```python
from build123d import *

# Parameters (mm, degrees)
F0_R     = 9
F0_R_2   = 9.5
F1_DEPTH = 3
F3_DEPTH = 6.001


with BuildPart() as f1:
    # F0 (on Top) → F1 (new body, symmetric)
    with BuildSketch(Plane.XY):
        with BuildLine():
            Line((22.5, 12.5), (-22.5, 12.5))
            ThreePointArc((-22.5, 12.5), (-31.338835, 8.838835), (-35, 0))
            ThreePointArc((-35, 0), (-31.338835, -8.838835), (-22.5, -12.5))
            Line((-22.5, -12.5), (22.5, -12.5))
            ThreePointArc((22.5, -12.5), (31.338835, -8.838835), (35, 0))
            ThreePointArc((35, 0), (31.338835, 8.838835), (22.5, 12.5))
        make_face()
        with Locations((-22.5, 0)):
            Circle(F0_R, mode=Mode.SUBTRACT)
        Circle(F0_R_2, mode=Mode.SUBTRACT)
        with Locations((22.5, 0)):
            Circle(F0_R, mode=Mode.SUBTRACT)
    extrude(amount=F1_DEPTH, both=True)

    # F2 (on face) → F3 (cut, through all)
    with BuildSketch(Plane.XY.offset(3)):
        with BuildLine():
            Line((22.5, 12.5), (0, 12.5))
            ThreePointArc((0, 12.5), (3.235238, 12.074073), (6.25, 10.825318))
            ThreePointArc((6.25, 10.825318), (11.25, 9.485572), (16.25, 10.825318))
            ThreePointArc((16.25, 10.825318), (19.264762, 12.074073), (22.5, 12.5))
        make_face()
        with BuildLine():
            ThreePointArc((-22.5, 12.5), (-19.264762, 12.074073), (-16.25, 10.825318))
            ThreePointArc((-16.25, 10.825318), (-11.25, 9.485572), (-6.25, 10.825318))
            ThreePointArc((-6.25, 10.825318), (-3.235238, 12.074073), (0, 12.5))
            Line((0, 12.5), (-22.5, 12.5))
        make_face()
        with BuildLine():
            ThreePointArc((6.25, -10.825318), (3.235238, -12.074073), (0, -12.5))
            Line((0, -12.5), (22.5, -12.5))
            ThreePointArc((22.5, -12.5), (19.264762, -12.074073), (16.25, -10.825318))
            ThreePointArc((16.25, -10.825318), (11.25, -9.485572), (6.25, -10.825318))
        make_face()
        with BuildLine():
            ThreePointArc((-16.25, -10.825318), (-19.264762, -12.074073), (-22.5, -12.5))
            Line((-22.5, -12.5), (0, -12.5))
            ThreePointArc((0, -12.5), (-3.235238, -12.074073), (-6.25, -10.825318))
            ThreePointArc((-6.25, -10.825318), (-11.25, -9.485572), (-16.25, -10.825318))
        make_face()
    extrude(amount=-F3_DEPTH, mode=Mode.SUBTRACT)


solid = f1.part
```
The listing builds one solid part. Answer for the finished solid, in the listing's coordinates (mm). Give positions to 0.01 mm unless a question says otherwise; leave off trailing zeros. Write each loop counter-clockwise with the first axis right and the second up, starting at its lowest first coordinate (ties: lowest second). Pieces come first, ordered by that corner, then holes. Notation, with made-up numbers: (83, 55) -> (96, 55) arc R12 cw to (96, 73) -> close; hole circle Ø8 at (85.25, 65). An arc over 180 degrees is marked (long way). Write item = value, one per line. Start each with the question number.
1) The part is cut by section C-C, the plane y = -6.5. Determine the outline of the cut face in (x, z), and give its area (3 significant figures).
2) This flat-tipped pin is pushed along its axis until it touches: pin 1 (1 mm diameter, centred on y = 5.5, z = -0.5, fed in from +X). Where does it stop, or does it pass through?
3) The part is cut by section A-A, the plane z = -1.45. Determine the outline of the cut face in (x, y), and give its area (3 significant figures).
4) Determine the mould class of faces 1 (the face through (-11.323, 9.486, 0.042)), 2 (the face through (-7.94, -5.5, -3)), 3 (the face through (31.084, 2.703, -0.042)) for opening direction Y: +Y half, -Y half, draft (parallel to the pull), parting line (faces both ways), or undercut.
5) The part is cut by section D-D, the plane x = -28. Determine the outline of the cut face in (y, z).
6) Straight lines are drawn through the part: line 1 along X through (y, z) = (-0.5, -0.45); line 2 along X through (y, z) = (3.75, -1.2); line 3 along X through (y, z) = (-11.5, 1.85). For each, find the intervals that lie inside material, in ascending order.
7) The part is cut by section B-B, the plane x = 26. Determine the outline of the cut face in (y, z), and give its area (3 significant figures).
Solutions:
q1.outline = (-33.18, -3) -> (-28.72, -3) -> (-28.72, 3) -> (-33.18, 3) -> close; (-16.28, -3) -> (-6.93, -3) -> (-6.93, 3) -> (-16.28, 3) -> close; (6.93, -3) -> (16.28, -3) -> (16.28, 3) -> (6.93, 3) -> close; (28.72, -3) -> (33.18, -3) -> (33.18, 3) -> (28.72, 3) -> close
q1.area = 166 mm²
q2.pin_1 = 33.96
q3.outline = (-35, 0) arc R12.5 ccw to (-22.5, -12.5) arc R12.5 ccw to (-16.25, -10.83) arc R10 cw to (-6.25, -10.83) arc R12.5 ccw to (6.25, -10.83) arc R10 cw to (16.25, -10.83) arc R12.5 ccw to (22.5, -12.5) arc R12.5 ccw to (35, 0) arc R12.5 ccw to (22.5, 12.5) arc R12.5 ccw to (16.25, 10.83) arc R10 cw to (6.25, 10.83) arc R12.5 ccw to (-6.25, 10.83) arc R10 cw to (-16.25, 10.83) arc R12.5 ccw to (-22.5, 12.5) arc R12.5 ccw to start; hole circle Ø18 at (-22.5, 0); hole circle Ø19 at (0, 0); hole circle Ø18 at (22.5, 0)
q3.area = 693 mm²
q4.face_1 = +Y half
q4.face_2 = draft
q4.face_3 = undercut
q5.outline = (-11.22, -3) -> (-7.12, -3) -> (-7.12, 3) -> (-11.22, 3) -> close; (7.12, -3) -> (11.22, -3) -> (11.22, 3) -> (7.12, 3) -> close
q6.line_1 = -34.99 to -31.49, -13.51 to -9.49, 9.49 to 13.51, 31.49 to 34.99
q6.line_2 = -34.42 to -30.68, -14.32 to -8.73, 8.73 to 14.32, 30.68 to 34.42
q6.line_3 = -27.4 to -17.6, -4.9 to 4.9, 17.6 to 27.4
q7.outline = (-12, -3) -> (-8.29, -3) -> (-8.29, 3) -> (-12, 3) -> close; (8.29, -3) -> (12, -3) -> (12, 3) -> (8.29, 3) -> close
q7.area = 44.5 mm²
